Autodesk Inventor part; units mm, degrees
ref_plane "YZ Plane" through (0, 0, 0) normal (1, 0, 0) x (0, 1, 0)
ref_plane "XZ Plane" through (0, 0, 0) normal (0, 1, 0) x (-1, 0, 0)
ref_plane "XY Plane" through (0, 0, 0) normal (0, 0, 1) x (1, 0, 0)
sketch "Sketch1" plane through (0, 0, 0) normal (0, 0, 1) x (1, 0, 0)
  circle A0 centre (0, 0) radius 3
  line L0 (-2.8868, 5) -> (2.8868, 5)
  line L1 (2.8868, 5) -> (5.7735, 0)
  line L2 (5.7735, 0) -> (2.8868, -5)
  line L3 (2.8868, -5) -> (-2.8868, -5)
  line L4 (-2.8868, -5) -> (-5.7735, 0)
  line L5 (-5.7735, 0) -> (-2.8868, 5)
  dimension "d0" = 6
  dimension "d1" = 10
extrude "Extrusion1" add sketch "Sketch1" along normal mid plane 4.5
sketch "Sketch2" plane through (0, 0, 2.25) normal (0, 0, 1) x (1, 0, 0)
  circle A0 centre (0, 0) radius 3
  circle A1 centre (0, 0) radius 4.6
  dimension "d6" = 9.2
extrude "Extrusion2" add sketch "Sketch2" along normal blind 1.5
sketch "Sketch4" plane through (0, 0, 0) normal (0, 1, 0) x (-1, 0, 0)
  line L0 (-2.8868, 2.25) -> (-5.7735, 2.25)
  line L1 (-5.7735, 2.25) -> (-5.7735, -2.25)
  line L2 (-5.7735, -2.25) -> (-2.8868, -2.25)
  line L3 (-2.8868, 2.25) -> (-2.8868, -2.25)
  line L4 (-4.6735, 2.25) -> (-5.7735, 1.6149)
  line L5 (-5.7735, -1.6149) -> (-4.6735, -2.25)
  line L6 (0, -3.5) -> (0, 3.5)
  dimension "d7" = 1.1
  dimension "d8" = 1.1
  dimension "d9" = 30
  dimension "d10" = 30
revolve "Revolution1" cut sketch "Sketch4" angle 360 about axis through (0, 0, -10) along (0, 0, 1) contours L4 L1 L0 | L2 L1 L5
fillet "Fillet1" radius 0.5 1 edges at (-4.6, 0, 3.75)
properties part number "M6 K-Nut Short" material "Steel"
Input: part model. Units: mm. Frame: model coordinates. A direction names the side the tool comes from. Round coordinates to 2 decimals unless told otherwise and drop trailing zeros. Loops run counter-clockwise (first coordinate to the right, second up) from the corner with the lowest first, then second, coordinate; pieces in that order, holes last. Notation, with made-up numbers: (-7.75, 56.5) - (43.25, 56.5) arc R19 cw to (43.25, 67.5) - close; hole circle Ø11 at (57, -30.75). An arc over 180 degrees is marked (long way). One line per item, written item: value. Start each with the question number.
(1) Section A-A, the plane x = 0. Return loops of the section in (y, z), plus the area to 3 significant figures.
(2) Draft query along Y for faces 1 (the flat face through (4.31, 2.535, -0.029)), 2 (the flat face through (-4.31, -2.535, -0.029)), 3 (the cylindrical face through (-3, 0, 1)), 4 (the flat face through (3, -1, -2.25)). Return one class per face: +Y half, -Y half, draft (parallel to the pull), parting line (faces both ways), or undercut.
(3) Ray query, line 1 (Y direction, x = 0, z = 0.9); line 2 (X direction, y = -0.25, z = -0.65); line 3 (Y direction, x = -1, z = 3.15). Return the intervals inside material, ascending. Write a range as [from, to].
(4) Section B-B, the plane z = 1.8. Return loops of the section in (x, y), plus the area to 3 significant figures.
(5) Section C-C, the plane z = 0.2. Return loops of the section in (x, y), plus the area to 3 significant figures.
(6) Access query for faces 5 (the cylindrical face through (-3.65, 2.8, 2.74)), 6 (the flat face through (0, 5, 0)). Directions: +Z, -Z, +X, -X, +Y, -Y. A direction counts if a zero-diameter tool reaches every point of the face in a straight line with its end or side. Return the directions, or none.
(7) Contact query for flat-ended pins moving along their axis: P1, Ø2, axis at y = 1, z = 2, coming from the +X side; P2, Ø4, axis at x = 3.5, y = 3.5, coming from the -Z side. Output: stop coordinate, or through.
Results below:
1. outline: (-5, -2.06) - (-4.67, -2.25) - (-3, -2.25) - (-3, 3.75) - (-4.1, 3.75) arc R0.5 ccw to (-4.6, 3.25) - (-4.6, 2.25) - (-4.67, 2.25) - (-5, 2.06) - close; (3, -2.25) - (4.67, -2.25) - (5, -2.06) - (5, 2.06) - (4.67, 2.25) - (4.6, 2.25) - (4.6, 3.25) arc R0.5 ccw to (4.1, 3.75) - (3, 3.75) - close
1. area: 22.6 mm^2
2. face 1: +Y half
2. face 2: -Y half
2. face 3: undercut
2. face 4: draft
3. line 1: [-5, -3], [3, 5]
3. line 2: [-5.63, -2.99], [2.99, 5.63]
3. line 3: [-4.49, -2.83], [2.83, 4.49]
4. outline: (-5.42, -0.62) - (-3.24, -4.38) arc R5.45 ccw to (-2.18, -5) - (2.18, -5) arc R5.45 ccw to (3.24, -4.38) - (5.42, -0.62) arc R5.45 ccw to (5.42, 0.62) - (3.24, 4.38) arc R5.45 ccw to (2.18, 5) - (-2.18, 5) arc R5.45 ccw to (-3.24, 4.38) - (-5.42, 0.62) arc R5.45 ccw to start; hole circle Ø6 at (0, 0)
4. area: 57.2 mm^2
5. outline: (-5.77, 0) - (-2.89, -5) - (2.89, -5) - (5.77, 0) - (2.89, 5) - (-2.89, 5) - close; hole circle Ø6 at (0, 0)
5. area: 58.3 mm^2
6. face 5: +Z
6. face 6: +Z, -Z, +X, -X, +Y
7. P1: x = 5.73
7. P2: z = -2.25
